from build123d import *

# Parameters (mm, degrees)
SKETCH1_R           = 1.5
SKETCH1_R_2         = 4.75
SKETCH1_R_3         = 1.75
BOSS_EXTRUDE1_DEPTH = 5


with BuildPart() as part:
    # Sketch1 → Boss-Extrude1 (new body)
    with BuildSketch(Plane.XY):
        with BuildLine():
            Line((-228.983312247, -100.327673659), (-31.823690309, -11.677627043))
            ThreePointArc((-31.823690309, -11.677627043), (-31.180096404, -11.740933542), (-30.549947196, -11.595562287))
            add(Edge.make_bspline(
                [(-7.332121112, -8.2), (-15.261701169, -7.378248506), (-23.028748322, -8.511718389), (-30.549947196, -11.595562287)],
                knots=[0, 0, 0, 0, 0.928485629, 0.928485629, 0.928485629, 0.928485629], degree=3))
            ThreePointArc((-7.332121112, -8.2), (10.276186063, -3.924283374), (0, 11))
            add(Edge.make_bspline(
                [(-37.223327458, -0.160922187), (-34.733241197, 1.803007777), (-22.33190483, 6.92754021), (-10.110124034, 10.988248808), (0, 11)],
                knots=[0.039876476, 0.039876476, 0.039876476, 0.039876476, 0.276467277, 1, 1, 1, 1], degree=3))
            Line((-37.223327458, -0.160922187), (-234.014760878, -88.645418023))
            add(Edge.make_bspline(
                [(-234.014760878, -88.645418023), (-237.136414749, -89.204727957), (-249.199971308, -95.080489992), (-260.348583277, -101.527949282), (-267.06700619, -109.08291716)],
                knots=[0.039876476, 0.039876476, 0.039876476, 0.039876476, 0.276467277, 1, 1, 1, 1], degree=3))
            ThreePointArc((-267.06700619, -109.08291716), (-262.722901285, -126.674477262), (-247.838660732, -116.340377524))
            add(Edge.make_bspline(
                [(-247.838660732, -116.340377524), (-243.190858822, -109.863383406), (-237.188340902, -104.805562326), (-229.890025639, -101.226020455)],
                knots=[0, 0, 0, 0, 0.928485629, 0.928485629, 0.928485629, 0.928485629], degree=3))
            ThreePointArc((-229.890025639, -101.226020455), (-229.363080717, -100.851120634), (-228.983312247, -100.327673659))
        make_face()
        with Locations((-8.2, 0)):
            Circle(SKETCH1_R, mode=Mode.SUBTRACT)
        with Locations((0, 8.2)):
            Circle(SKETCH1_R, mode=Mode.SUBTRACT)
        with Locations((0, -8.2)):
            Circle(SKETCH1_R, mode=Mode.SUBTRACT)
        with Locations((8.2, 0)):
            Circle(SKETCH1_R, mode=Mode.SUBTRACT)
        Circle(SKETCH1_R_2, mode=Mode.SUBTRACT)
        with Locations(Location((-258.838577689, -116.383120199, 0), (0, 0, 180))):
            Circle(SKETCH1_R_2, mode=Mode.SUBTRACT)
        with Locations(Location((-264.280547227, -122.517039627, 0), (0, 0, 180))):
            Circle(SKETCH1_R, mode=Mode.SUBTRACT)
        with Locations(Location((-252.704658261, -121.825089736, 0), (0, 0, 180))):
            Circle(SKETCH1_R, mode=Mode.SUBTRACT)
        with Locations(Location((-264.972497117, -110.941150661, 0), (0, 0, 180))):
            Circle(SKETCH1_R, mode=Mode.SUBTRACT)
        with Locations(Location((-253.396608151, -110.249200771, 0), (0, 0, 180))):
            Circle(SKETCH1_R, mode=Mode.SUBTRACT)
        with Locations((-75.674055251, -25.316000748)):
            Circle(SKETCH1_R_3, mode=Mode.SUBTRACT)
        with Locations((-30.071768827, -4.811575057)):
            Circle(SKETCH1_R_3, mode=Mode.SUBTRACT)
        with Locations((-121.276341675, -45.820426439)):
            Circle(SKETCH1_R_3, mode=Mode.SUBTRACT)
        with Locations(Location((-235.282057735, -97.081490667, 0), (0, 0, 180))):
            Circle(SKETCH1_R_3, mode=Mode.SUBTRACT)
        with Locations(Location((-189.679771311, -76.577064976, 0), (0, 0, 180))):
            Circle(SKETCH1_R_3, mode=Mode.SUBTRACT)
        with Locations(Location((-144.077484887, -56.072639285, 0), (0, 0, 180))):
            Circle(SKETCH1_R_3, mode=Mode.SUBTRACT)
    extrude(amount=BOSS_EXTRUDE1_DEPTH)


solid = part.part
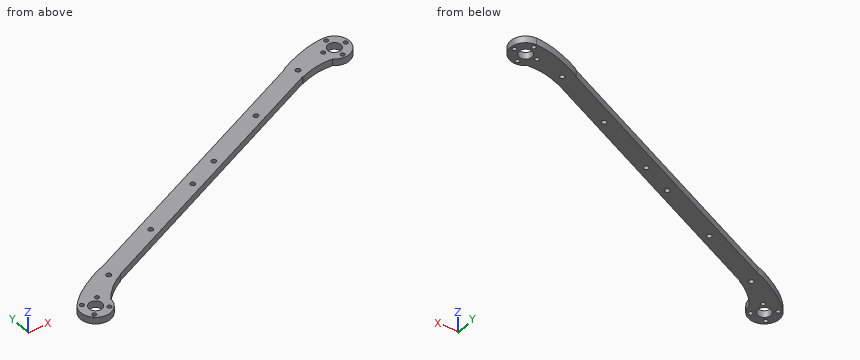
Geometry: final body of the model. Coordinates: model frame, mm. Coordinates: 2 decimals unless noted, no trailing zeros. Loops run counter-clockwise (first coordinate to the right, second up) from the corner with the lowest first, then second, coordinate; pieces in that order, holes last. Notation, with made-up numbers: M 60.25,6.5 L 69.25,6.5 A24 cw 69.25,26.5 Z; hole C -32.75,67 d11. An arc over 180 degrees is marked long. One line per item, written item: value. Start each with the question number.
1) Pin query (flat end, axial travel): P1, Ø1.5, axis at y = -13.5, z = 4, coming from the +X side; P2, Ø3, axis at y = -27, z = 1.5, coming from the -X side; P3, Ø1.5, axis at x = -163, z = 2, coming from the +Y side. Return the tip coordinate at first contact, or that it passes through.
2) Material intervals for L1, parallel to X at y = -110, z = 2.25; L2, parallel to X at y = -116, z = 3; L3, parallel to X at y = -115, z = 3.35, sorted ascending. Write a range as from..to.
3) Cut plane A-A (y = -72). Return loops of the section in (x, z) (3 decimals).
4) Cut plane C-C (z = 2.85). Count the separate pieces of the cut face and the enclosed holes in it, then the cut area to 3 significant figures.
5) Cut plane B-B (x = -216.5). Return loops of the section in (y, z).
Evaluation:
1. P1: x = -34.21
1. P2: x = -100.25
1. P3: y = -56.38
2. L1: -267.8..-266.14, -263.8..-254.88, -251.92..-242.4
2. L2: -269.83..-263.57, -254.1..-247.59
2. L3: -269.75..-263.38, -254.29..-246.84
3. outline: M -196.995,0 L -165.982,0 L -165.982,5 L -196.995,5 Z
4. separate pieces: 1
4. enclosed holes: 16
4. area: 4,060 mm^2
5. outline: M -94.71,0 L -80.77,0 L -80.77,5 L -94.71,5 Z
